The listing builds one solid part. Answer for the finished solid, in the listing's coordinates (mm). Give positions to 0.01 mm unless a question says otherwise; leave off trailing zeros. Write each loop counter-clockwise with the first axis right and the second up, starting at its lowest first coordinate (ties: lowest second). Pieces come first, ordered by that corner, then holes.
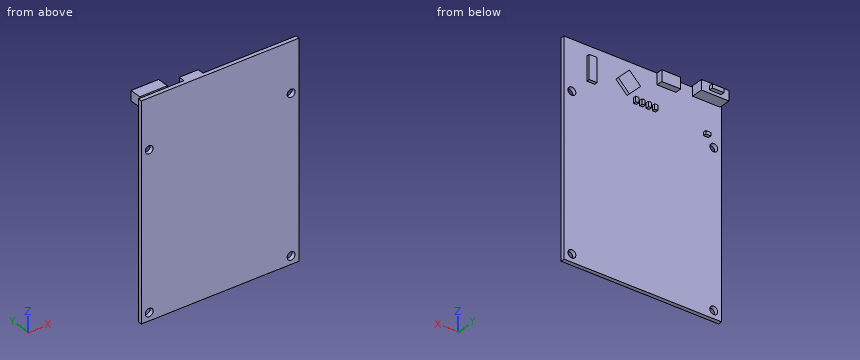
```python
from build123d import *

# Parameters (mm, degrees)
SKETCH1_W                = 63.5
SKETCH1_H                = 84.455
SKETCH1_R                = 1.5875
BOSS_EXTRUDE1_DEPTH      = 1.6
SKETCH2_W                = 1.27
SKETCH2_H                = 2.032
SKETCH2_W_2              = 3.175
SKETCH2_H_2              = 9.525
SKETCH2_W_3              = 2.032
SKETCH2_H_3              = 1.27
BOSS_EXTRUDE2_DEPTH      = 1.27
SKETCH3_W                = 7.62
SKETCH3_H                = 4.445
BOSS_EXTRUDE3_DEPTH      = 2.54
BOSS_EXTRUDE4_DEPTH      = 1.984375
BOSS_EXTRUDE4_DEPTH_BACK = 1.984375
BOSS_EXTRUDE4_START      = -1.42875
SKETCH4_W                = 4.7625
SKETCH4_H                = 1.5875
CUT_EXTRUDE1_REACH       = 94.284
CUT_EXTRUDE1_START       = -1.190625
SKETCH5_W                = 4.7625
SKETCH5_H                = 1.5875
CUT_EXTRUDE2_REACH       = 95.872
CUT_EXTRUDE2_START       = -2.778125
SKETCH5_2_W              = 4.7625
SKETCH5_2_H              = 1.5875


with BuildPart() as part:
    # Sketch1 → Boss-Extrude1 (new body)
    with BuildSketch(Plane(origin=(0, 0, 0), x_dir=(1, 0, 0), z_dir=(0, 1, 0))):
        Rectangle(SKETCH1_W, SKETCH1_H)
        with Locations(Location((-28.575, 39.0525, 0), (0, 0, 270))):
            Circle(SKETCH1_R, mode=Mode.SUBTRACT)
        with Locations(Location((28.575, 39.0525, 0), (0, 0, 270))):
            Circle(SKETCH1_R, mode=Mode.SUBTRACT)
        with Locations(Location((-28.575, -22.5425, 0), (0, 0, 270))):
            Circle(SKETCH1_R, mode=Mode.SUBTRACT)
        with Locations(Location((28.575, -22.5425, 0), (0, 0, 270))):
            Circle(SKETCH1_R, mode=Mode.SUBTRACT)
    extrude(amount=BOSS_EXTRUDE1_DEPTH)

    # Sketch2 → Boss-Extrude2 (add)
    with BuildSketch(Plane(origin=(0, 1.6, 0), x_dir=(1, 0, 0), z_dir=(0, 1, 0))):
        Polygon((6.35, -29.228371939), (10.840128061, -33.7185), (6.35, -38.208628061), (1.859871939, -33.7185), align=None)
        with Locations((-1.905, -28.2575)):
            Rectangle(SKETCH2_W, SKETCH2_H)
        with Locations((-4.445, -28.2575)):
            Rectangle(SKETCH2_W, SKETCH2_H)
        with Locations((0.635, -28.2575)):
            Rectangle(SKETCH2_W, SKETCH2_H)
        with Locations((3.175, -28.2575)):
            Rectangle(SKETCH2_W, SKETCH2_H)
        with Locations((20.955, -33.3375)):
            Rectangle(SKETCH2_W_2, SKETCH2_H_2)
        with Locations((-25.4, -26.19375)):
            Rectangle(SKETCH2_W_3, SKETCH2_H_3)
    extrude(amount=BOSS_EXTRUDE2_DEPTH)

    # Sketch3 → Boss-Extrude3 (add)
    with BuildSketch(Plane(origin=(0, 1.6, 0), x_dir=(1, 0, 0), z_dir=(0, 1, 0))):
        with Locations((-9.525, -40.005)):
            Rectangle(SKETCH3_W, SKETCH3_H)
    extrude(amount=BOSS_EXTRUDE3_DEPTH)

    # Sketch4 → Boss-Extrude4 (add, two sides: drawn at the far end of the back side and taken through both)
    with BuildSketch(Plane.XY.offset(42.2275).offset(BOSS_EXTRUDE4_START - BOSS_EXTRUDE4_DEPTH_BACK)):
        with Locations((-25.55875, 7.15625)):
            Rectangle(SKETCH4_W, SKETCH4_H)
        Polygon((-27.94, 6.3625), (-31.115, 6.3625), (-31.115, 1.6), (-20.0025, 1.6), (-20.0025, 6.3625), (-23.1775, 6.3625), align=None)
    extrude(amount=BOSS_EXTRUDE4_DEPTH + BOSS_EXTRUDE4_DEPTH_BACK)

    # Sketch5 → Cut-Extrude1 (cut, up to next)
    with BuildSketch(Plane.XY.offset(42.783125).offset(CUT_EXTRUDE1_START), mode=Mode.PRIVATE) as cut_extrude1_sk1:
        with Locations((-25.55875, 7.15625)):
            Rectangle(SKETCH5_W, SKETCH5_H)
    cut_extrude1_tool1 = extrude(cut_extrude1_sk1.sketch, amount=CUT_EXTRUDE1_REACH, mode=Mode.PRIVATE) & part.part
    add(cut_extrude1_tool1.solids().sort_by_distance((-25.55875, 7.15625, 41.5925))[0], mode=Mode.SUBTRACT)

    # Sketch5_2 → Cut-Extrude2 (cut, up to next)
    with BuildSketch(Plane.XY.offset(42.783125).offset(CUT_EXTRUDE2_START), mode=Mode.PRIVATE) as cut_extrude2_sk1:
        with Locations((-25.55875, 7.15625)):
            Rectangle(SKETCH5_2_W, SKETCH5_2_H)
    cut_extrude2_tool1 = extrude(cut_extrude2_sk1.sketch, amount=-CUT_EXTRUDE2_REACH, mode=Mode.PRIVATE) & part.part
    add(cut_extrude2_tool1.solids().sort_by_distance((-25.55875, 7.15625, 40.005))[0], mode=Mode.SUBTRACT)


solid = part.part
```
Item 1: A cutting plane is placed at D-D, the plane y = 5.5. Give the vertices of the cut face in (x, z) (1 decimal).
Conclusion:
outline: (-31.1, 38.8) - (-20, 38.8) - (-20, 42.8) - (-31.1, 42.8) - close
Item 2: Each of these flat-tipped pins is pushed along its axis until it touches: P1, Ø3.5, axis at x = -8, z = 41, coming from the +Y side; P2, Ø1.7, axis at x = -25, y = 7.5, coming from the +Z side; P3, Ø4, axis at x = -28.58, z = 22.54, coming from the +Y side. Where does it stop, or does it pass through?
Conclusion:
P1: stops at y = 4.14
P2: stops at z = 41.59
P3: stops at y = 1.6
Item 3: Consider probe 1 along Y at (x, z) = (-27.5, -22.5); probe 2 along Z at (x, y) = (28, 1.5); probe 3 along X at (y, z) = (5.5, 39) (1 decimal). Determine where each line is inside the solid, lowest interval first.
Conclusion:
probe 1: y = 0 to 1.6
probe 2: z = -42.23 to -40.53, -37.57 to 21.06, 24.02 to 42.23
probe 3: x = -31.1 to -20
Item 4: A cutting plane is placed at B-B, the plane z = -1.5. Give the vertices of the cut face in (x, y).
Conclusion:
outline: (-31.75, 0) - (31.75, 0) - (31.75, 1.6) - (-31.75, 1.6) - close
Item 5: A cutting plane is placed at C-C, the plane x = -11.5. Give the vertices of the cut face in (y, z).
Conclusion:
outline: (0, -42.23) - (1.6, -42.23) - (1.6, 37.78) - (4.14, 37.78) - (4.14, 42.23) - (0, 42.23) - close
Item 6: A cutting plane is placed at A-A, the plane x = 21.5. Give the vertices of the cut face in (y, z) (1 decimal), plus the area to 3 significant figures.
Conclusion:
outline: (0, -42.2) - (1.6, -42.2) - (1.6, 28.6) - (2.9, 28.6) - (2.9, 38.1) - (1.6, 38.1) - (1.6, 42.2) - (0, 42.2) - close
area: 147 mm2
